Autodesk Fusion 360 part; units mm, degrees
sketch "Sketch1" plane through (0, 0, 0) normal (0, 1, 0) x (1, 0, 0)
  line L0 (190, -75) -> (-190, -75)
  line L1 (-190, -75) -> (-190, 75)
  line L2 (-190, 75) -> (190, 75)
  line L3 (190, 75) -> (190, -75)
  line L4 (190, -75) -> (-190, 75) construction
  line L5 (-190, -75) -> (190, 75) construction
  dimension "d1" = 380
  dimension "d2" = 150
extrude "Extrude1" add sketch "Sketch1" along normal blind 20
sketch "Sketch2" plane through (0, 20, 0) normal (0, 1, 0) x (-1, 0, 0)
  line L0 (-190, -75) -> (190, -75)
  line L1 (190, -75) -> (190, 75)
  line L2 (190, 75) -> (-190, 75)
  line L3 (-190, 75) -> (-190, -75)
  circle A0 centre (0, 0) radius 75
  line L4 (0, 0) -> (-150, 0)
  line L5 (0, 0) -> (150, 0)
  circle A1 centre (150, 0) radius 40
  circle A2 centre (-150, 0) radius 40
  line L6 (190, 0) -> (175, 0)
  line L7 (175, 0) -> (175, -10)
  line L8 (175, -10) -> (188.7298, -10)
  line L9 (175, 0) -> (175, 10)
  line L10 (175, 10) -> (188.7298, 10)
  line L11 (-190, 0) -> (-175, 0)
  line L12 (-175, 0) -> (-175, -10)
  line L13 (-175, 0) -> (-175, 10)
  line L14 (-175, -10) -> (-188.7298, -10)
  line L15 (-175, 10) -> (-188.7298, 10)
  line L16 (-188.7298, -10) -> (-190, -10)
  line L17 (-188.7298, 10) -> (-190, 10)
  line L18 (188.7298, -10) -> (190, -10)
  line L19 (188.7298, 10) -> (190, 10)
  circle A3 centre (150, 0) radius 25
  line L20 (175, -10) -> (172.9129, -10)
  line L21 (172.9129, 10) -> (175, 10)
  line L22 (172.9129, 10) -> (172.9129, -10)
  circle A4 centre (-150, 0) radius 25
  line L23 (-175, -10) -> (-172.9129, -10)
  line L24 (-172.9129, -10) -> (-172.9129, 10)
  line L25 (-172.9129, 10) -> (-175, 10)
  line L26 (-190, 10) -> (-190, -10)
  line L27 (-188.7298, -10) -> (-190, -10)
  line L28 (-188.7298, 10) -> (-190, 10)
  line L29 (0, -75) -> (-190, -75)
  line L30 (0, -75) -> (0, 75)
  line L31 (-190, 75) -> (-190, -75)
  line L32 (-150, 0) -> (-150, -75)
  line L33 (-150, 0) -> (-150, 75)
  line L34 (0, 75) -> (-150, 75)
  line L35 (150, 0) -> (150, 75)
  line L36 (0, 75) -> (150, 75)
  line L37 (150, 0) -> (150, -75)
  line L38 (150, -75) -> (0, -75)
  arc A5 (150, -40) -> (44.1171, -60.6521) centre (150, -321.7554) ccw
  arc A6 (-44.1171, -60.6521) -> (-150, -40) centre (-150, -321.7554) ccw
  arc A7 (-150, 40) -> (-44.1171, 60.6521) centre (-150, 321.7554) ccw
  arc A8 (44.1171, 60.6521) -> (150, 40) centre (150, 321.7554) ccw
  dimension "d5" = 150
  dimension "d6" = 150
  dimension "d7" = 80
  dimension "d19" = 15
  dimension "d20" = 10
  dimension "d21" = 10
  dimension "d22" = 15
  dimension "d23" = 10
  dimension "d24" = 10
hole "Hole1" at (0, 20, 0) direction (0, -1, 0) diameter 100 depth 20 tip angle 180 counterbore diameter 135.6 counterbore depth 10
hole "Hole2" at (-150, 20, 0) direction (0, -1, 0) diameter 50 depth 20 tip angle 180
hole "Hole3" at (150, 20, 0) direction (0, -1, 0) diameter 50 depth 20 tip angle 180
extrude "Extrude2" cut sketch "Sketch2" against normal blind 20 contours A2 L11 L12 L14 | A2 L11 L13 L15 | A1 L6 L7 L8 | A1 L6 L9 L10
extrude "Extrude3" cut sketch "Sketch2" against normal blind 20 contours L1 A1 L18 | L1 A1 L19
extrude "Extrude4" cut sketch "Sketch2" against normal blind 20 contours L7 A3 L20 | L9 A3 L21
extrude "Extrude5" cut sketch "Sketch2" against normal blind 20 contours L12 A4 L23 | L13 A4 L25
extrude "Extrude6" cut sketch "Sketch2" against normal blind 20 contours L3 A2 L16 L26 L27 L31 | L3 A2 L17 L26 L28 L31
extrude "Extrude7" cut sketch "Sketch2" against normal blind 20 contours L0 L3 A2 L16 L27 L29 L31 L32 | L0 A0 L29 L32 A6 | L0 A0 L37 L38 A5 | L0 L1 A1 L18 L37 | L2 L3 A2 L17 L28 L31 L33 | L2 A0 L33 L34 A7 | L2 A0 L35 L36 A8 | L1 L2 A1 L19 L35
Verification items for the finished model (mm, model axes). A direction names the side the tool comes from. Give positions to 0.01 mm unless a question says otherwise; leave off trailing zeros. Order: outer loops, then holes, each group sorted by start corner. A loop starts at its lowest first (then second) coordinate and runs counter-clockwise, first axis right, second up. Notation, with made-up numbers: M 61.5,-30.75 L 107.5,-30.75 A19 ccw 107.5,1.25 Z; hole C 22,88.5 d6. An arc over 180 degrees is marked long. Return JSON: item names as keys, results as strings. Group by question number.
1) Access from +Z, -Z, +X, -X, +Y, -Y to the whole of each face (thin tool, end or side, straight path). Record for faces 1 (the face through (181, 10, 10)), 2 (the face through (-96.807, 10.14, -45.067)), 3 (the face through (-181, 10, 10)), 4 (the face through (50, 10, -5)).
2) Mould release check, pull along Z, two halves, no side actions. Record for faces 5 (the face through (95.315, 10.14, -45.358)), 6 (the face through (125.02, 9.86, 0.96)), 7 (the face through (-181, 10, -10)), 8 (the face through (-95.315, 10.14, 45.358)): pulls with the +Z half, pulls with the -Z half, needs draft (parallel to the pull), parting line crosses it, or undercut.
3) Section check A-A on x = 0. Record the cut outline in (y, z).
4) Go/stop test with flat-tipped pins: pin 1 Ø8 at (y, z) = (17, 25) entering from +X; pin 2 Ø8 at (x, y) = (179.5, 5) entering from +Z; pin 3 Ø1.5 at (y, z) = (4.5, 4) entering from -X. Record where each tip stops, or that it passes through.
5) Section check B-B on z = 0. Record the cut outline in (x, y), and give its area (3 significant figures).
6) Scan lines: line 1 (X direction, y = 14.25, z = 0); line 2 (Z direction, x = 150, y = 7.75); line 3 (Z direction, x = 0, y = 18). Record each from-to range of solid material in increasing order.
7) Section check D-D on x = 54. Record the cut outline in (y, z).
8) Section check C-C on y = 6.75. Record the cut outline in (x, z), and give its area (3 significant figures).
Answer block:
{
 "1": {"face 1": "+X, +Y, -Y", "face 2": "-Z, -X, +Y, -Y", "face 3": "-X, +Y, -Y", "face 4": "+Y"},
 "2": {"face 5": "pulls with the -Z half", "face 6": "undercut", "face 7": "undercut", "face 8": "pulls with the +Z half"},
 "3": {"outline": "M 0,-75 L 20,-75 L 20,-67.8 L 10,-67.8 L 10,-50 L 0,-50 Z; M 0,50 L 10,50 L 10,67.8 L 20,67.8 L 20,75 L 0,75 Z"},
 "4": {"pin 1": "stops at x = 184.04", "pin 2": "stops at z = 30.82", "pin 3": "stops at x = -125.46"},
 "5": {"outline": "M -125,0 L -50,0 L -50,10 L -67.8,10 L -67.8,20 L -125,20 Z; M 50,0 L 125,0 L 125,20 L 67.8,20 L 67.8,10 L 50,10 Z", "area": "2,640 mm^2"},
 "6": {"line 1": "x = -125 to -67.8, 67.8 to 125", "line 2": "z = -40 to -25, 25 to 40", "line 3": "z = -75 to -67.8, 67.8 to 75"},
 "7": {"outline": "M 0,-56.86 L 20,-56.86 L 20,-41 L 10,-41 L 10,41 L 20,41 L 20,56.86 L 0,56.86 Z"},
 "8": {"outline": "M -188.73,-10 A40 ccw -150,-40 A281.76 cw -44.12,-60.65 A75 ccw 44.12,-60.65 A281.76 cw 150,-40 A40 ccw 188.73,-10 L 172.91,-10 A25 cw long 172.91,10 L 188.73,10 A40 ccw 150,40 A281.76 cw 44.12,60.65 A75 ccw -44.12,60.65 A281.76 cw -150,40 A40 ccw -188.73,10 L -172.91,10 A25 cw long -172.91,-10 Z; hole C 0,0 d100", "area": "24,900 mm^2"}
}
